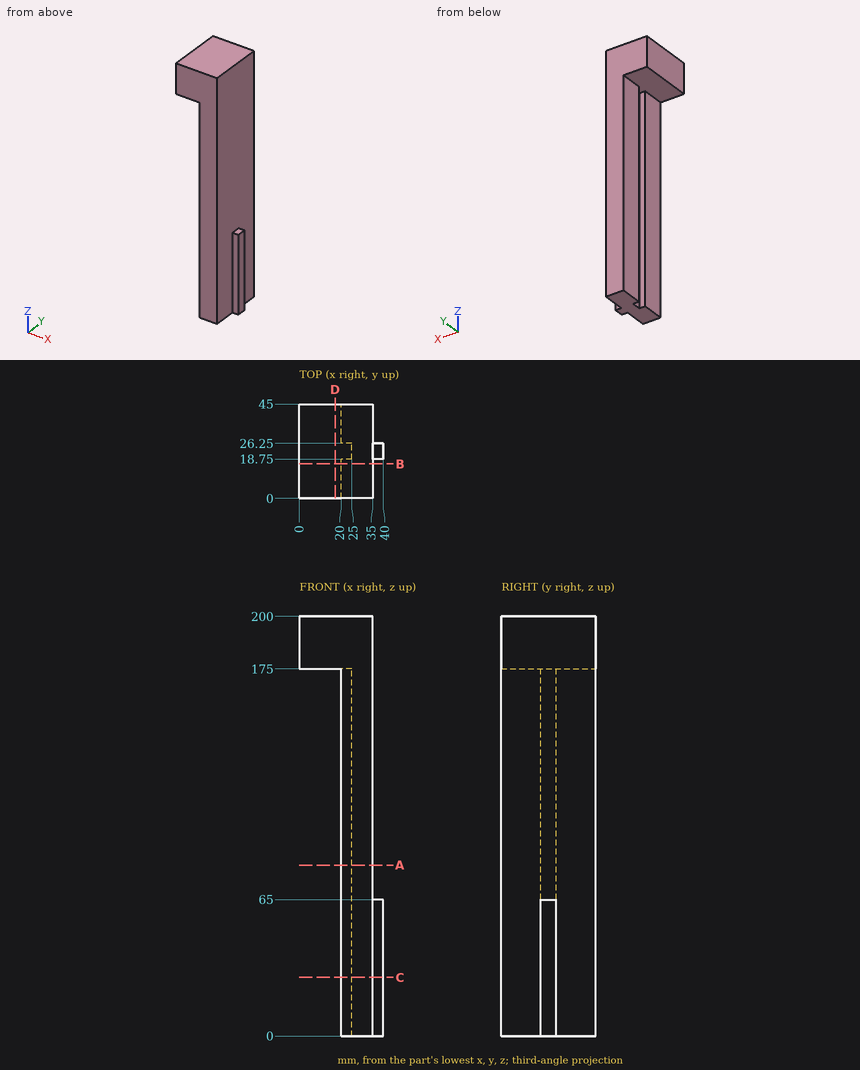
Geometry: see drawing. Coordinates: mm, zero at the bounding-box minimum. Coordinates: 2 decimals unless noted, no trailing zeros. Write each loop counter-clockwise with the first axis right and the second up, starting at its lowest first coordinate (ties: lowest second). Pieces come first, ordered by that corner, then holes. Notation, with made-up numbers: M 72,-6 L 130,-6 A9 cw 130,8 Z; hole C 21,-23 d11. An arc over 180 degrees is marked long. Use CSV: the item, a comma, the result in double quotes. Start each with the question number.
1. First-contact query: P1, Ø4, axis at x = 38, z = 22, coming from the +Y side; P2, Ø2, axis at y = 23.5, z = 116.5, coming from the -X side; P3, Ø10, axis at y = 20.5, z = 134.5, coming from the -X side. Flat tips, straight axial feed; report the tip coordinate or a pass-through.
2. Cut plane A-A on z = 81.5. Return the cut outline in (x, y), plus the area to 4 significant figures.
3. Cut plane D-D on x = 17. Return the cut outline in (y, z), plus the area to 4 significant figures.
4. Cut plane B-B on y = 16.5. Return the cut outline in (x, z), plus the area to 3 significant figures.
5. Ray query, probe 1 along Y at (x, z) = (21, 120.5); probe 2 along X at (y, z) = (16, 106); probe 3 along Z at (x, y) = (2, 30). Return the intervals inside material, ascending.
6. Cut plane C-C on z = 28. Return the cut outline in (x, y).
Entries:
1,P1,"y = 26.25"
1,P2,"x = 25"
1,P3,"x = 20"
2,outline,"M 20,0 L 35,0 L 35,45 L 20,45 L 20,26.25 L 25,26.25 L 25,18.75 L 20,18.75 Z"
2,area,"637.5 mm²"
3,outline,"M 0,175 L 45,175 L 45,200 L 0,200 Z"
3,area,"1,125 mm²"
4,outline,"M 0,175 L 20,175 L 20,0 L 35,0 L 35,200 L 0,200 Z"
4,area,"3,500 mm²"
5,probe 1,"0 to 18.75, 26.25 to 45"
5,probe 2,"20 to 35"
5,probe 3,"175 to 200"
6,outline,"M 20,0 L 35,0 L 35,18.75 L 40,18.75 L 40,26.25 L 35,26.25 L 35,45 L 20,45 L 20,26.25 L 25,26.25 L 25,18.75 L 20,18.75 Z"
